Source: CAD feature listing. Evaluate the final solid. Frame: model axes, mm. Coordinates: 2 decimals unless noted, no trailing zeros. Order: outer loops, then holes, each group sorted by start corner. A loop starts at its lowest first (then second) coordinate and runs counter-clockwise, first axis right, second up. Notation, with made-up numbers: (-26.5, -35.75) -> (14.5, -35.75) arc R21 cw to (14.5, -4.75) -> close; hole circle Ø5 at (-18, -20.5). An arc over 180 degrees is marked (long way). Write item = value, one per line. Start each with the question number.
Item 1: Section query B-B (x = 13). Count the separate pieces of the cut face and the enclosed holes in it, then the cut area to 3 significant figures.
Item 2: Mould query, pull axis Y, two halves, no side actions, for faces 1 (the flat face through (0, 0, -125)), 2 (the flat face through (0, 0, -120)). Classes: released by +Y, released by -Y, zero draft, split by the parting line, or undercut.
Item 3: Section query A-A (z = 37.5). Output: boundary loops of the cut face in (x, y) (3 decimals).
Item 4: Contact query for flat-ended pins moving along their axis: pin 1 (10 mm diameter, centred on y = -29.5, z = -0.5, fed in from -X); pin 2 (8 mm diameter, centred on x = -4.5, y = -23.5, fed in from +Z); pin 3 (4 mm diameter, centred on x = 24, z = -24, fed in from -Y). Output: stop coordinate, or through.
Item 5: Section query C-C (z = 65). Output: boundary loops of the cut face in (x, y).
Item 6: Ray query, line 1 along X through (y, z) = (-10, -17.5); line 2 along Z through (x, y) = (-14.5, 23.5); line 3 along Z through (x, y) = (3.5, 33). Return the intervals inside material, ascending. Write a range as [from, to].
```python
from build123d import *

# Parameters (mm, degrees)
F2_T = -5


with BuildPart() as f1:
    # F0 (on Front) → F1 (revolve)
    with BuildSketch(Plane.XZ):
        with BuildLine():
            Line((-25, -125), (0, -125))
            Line((0, -125), (0, 125))
            ThreePointArc((0, 125), (-18.2456196083, 115.4417277094), (-20.7752386162, 95))
            ThreePointArc((-20.7752386162, 95), (-14.7381173167, 46.1985321612), (-31.5822772233, 0))
            ThreePointArc((-31.5822772233, 0), (-48.9540387536, -63.5880714958), (-25, -125))
        make_face()
    revolve(axis=Axis((0, 0, 0), (0, 0, 1)))

    # F2 (hollow: no face is removed)
    offset(amount=F2_T, kind=Kind.INTERSECTION, mode=Mode.SUBTRACT)


solid = f1.part
```
Computed:
q1.separate_pieces = 1
q1.enclosed_holes = 2
q1.area = 3,540 mm^2
q2.face_1 = zero draft
q2.face_2 = undercut
q3.outline = circle Ø32.198 at (0, 0); hole circle Ø22.01 at (0, 0)
q4.pin_1 = -22.2
q4.pin_2 = 112.58
q4.pin_3 = -37.67
q5.outline = circle Ø28.59 at (0, 0); hole circle Ø18.57 at (0, 0)
q6.line_1 = [-39.71, -34.06], [34.06, 39.71]
q6.line_2 = [-121.71, -113.07], [-3.06, 6.48]
q6.line_3 = [-113.64, -103.49], [-12.64, -2.49]
